from build123d import *

# Parameters (mm, degrees)
SKETCH1_R           = 139.7
SKETCH1_R_2         = 14
BOSS_EXTRUDE1_DEPTH = 9.525
SKETCH2_R           = 2
CUT_EXTRUDE1_DEPTH  = 198.795110215
CIRPATTERN1_COUNT   = 6
CHAMFER1_SIZE       = 3


with BuildPart() as part:
    # Sketch1 → Boss-Extrude1 (new body)
    with BuildSketch(Plane.XY):
        with Locations(Location((0, 0, 0), (0, 0, 180))):
            Circle(SKETCH1_R)
        with Locations(Location((0, 0, 0), (0, 0, 180))):
            Circle(SKETCH1_R_2, mode=Mode.SUBTRACT)
    extrude(amount=BOSS_EXTRUDE1_DEPTH)

    # Sketch2 → Cut-Extrude1 (cut, through all)
    with BuildSketch(Plane.XY.offset(9.525)):
        with Locations((0, 25)):
            Circle(SKETCH2_R)
    cut_extrude1 = extrude(amount=-CUT_EXTRUDE1_DEPTH, mode=Mode.SUBTRACT)

    # CirPattern1: Cut-Extrude1 ×6 about axis
    cirpattern1_axis = Axis((0, 0, 0), (0, 0, 1))
    for i in range(1, CIRPATTERN1_COUNT):
        add(cut_extrude1.rotate(cirpattern1_axis, i * 360 / CIRPATTERN1_COUNT), mode=Mode.SUBTRACT)

    # Chamfer1
    chamfer1_edges = [part.edges().sort_by_distance(p)[0] for p in [
        (-2, 25, 9.525),
        (-22.650635095, 10.767949192, 9.525),
        (-20.650635095, -14.232050808, 9.525),
        (2, -25, 9.525),
        (22.650635095, -10.767949192, 9.525),
        (20.650635095, 14.232050808, 9.525),
    ]]
    chamfer(chamfer1_edges, length=CHAMFER1_SIZE)


solid = part.part
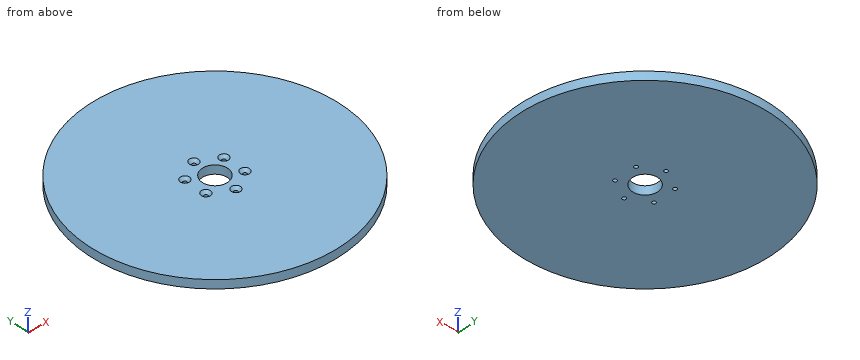
Design review of the part built by this model. Coordinates are the model's own, in mm. Give positions to 0.01 mm unless a question says otherwise; leave off trailing zeros. Loops run counter-clockwise (first coordinate to the right, second up) from the corner with the lowest first, then second, coordinate; pieces in that order, holes last. Notation, with made-up numbers: (57, 41) -> (79, 41) arc R28 ccw to (79, 63) -> close; hole circle Ø9 at (-26, 20.25). An arc over 180 degrees is marked (long way). One line per question, with ' | ' between items. Start each with the question number.
(1) We need section C-C (y = 38). State the section outline as (x, z) points (3 decimals), and give its area (3 significant figures).
(2) We need section B-B (x = 34). State the section outline as (y, z) points (3 decimals).
(3) Insertion check: P1, Ø17, axis at x = 0, y = 0, coming from the +Z side; P2, Ø6.5, axis at x = 21.65, y = -12.5, coming from the +Z side; P3, Ø1, axis at x = 78, z = 3, coming from the -Y side; P4, Ø1.5, axis at x = -70, z = 3, coming from the -Y side. Each pin has a flat end and moves straight along its axis. Give the tip position at first contact, or say it passes through.
(4) We need section A-A (z = 2.5). State the section outline as (x, y) points.
(5) For line 1 (Y direction, x = 0, z = 4.25); line 2 (Y direction, x = -1, z = 2.5); line 3 (X direction, y = -25, z = 4.5), list the stretches that pass through material, from the lowest coordinate up.
The answers:
1) outline: (-134.432, 0) -> (134.432, 0) -> (134.432, 9.525) -> (-134.432, 9.525) -> close | area: 2,560 mm^2
2) outline: (-135.499, 0) -> (135.499, 0) -> (135.499, 9.525) -> (-135.499, 9.525) -> close
3) P1: passes through | P2: stops at z = 7.78 | P3: stops at y = -116.23 | P4: stops at y = -121.33
4) outline: circle Ø279.4 at (0, 0); hole circle Ø4 at (-21.65, -12.5); hole circle Ø4 at (-21.65, 12.5); hole circle Ø28 at (0, 0); hole circle Ø4 at (0, -25); hole circle Ø4 at (0, 25); hole circle Ø4 at (21.65, -12.5); hole circle Ø4 at (21.65, 12.5)
5) line 1: y = -139.7 to -27, -23 to -14, 14 to 23, 27 to 139.7 | line 2: y = -139.7 to -26.73, -23.27 to -13.96, 13.96 to 23.27, 26.73 to 139.7 | line 3: x = -137.44 to -2, 2 to 137.44
